```python
from build123d import *

# Parameters (mm, degrees)
SKETCH2_W           = 6.5
SKETCH2_H           = 6.5
BOSS_EXTRUDE1_DEPTH = 8.5
SKETCH4_W           = 15
SKETCH4_H           = 2
BOSS_EXTRUDE2_DEPTH = 15
SKETCH5_R           = 2.7
CUT_EXTRUDE1_DEPTH  = 23.774998804
SKETCH6_W           = 6.5
SKETCH6_H           = 87
BOSS_EXTRUDE3_DEPTH = 2
CUT_EXTRUDE3_DEPTH  = 103.034534305
CUT_EXTRUDE4_DEPTH  = 99.257059971
CUT_EXTRUDE5_DEPTH  = 99.257059971
CUT_EXTRUDE6_DEPTH  = 99.257059971
CUT_EXTRUDE7_DEPTH  = 103.034534305


with BuildPart() as part:
    # Sketch2 → Boss-Extrude1 (new body)
    with BuildSketch(Plane(origin=(0, 0, 0), x_dir=(1, 0, 0), z_dir=(0, 1, 0))):
        with Locations((-0.156417112, 0.017379679)):
            Rectangle(SKETCH2_W, SKETCH2_H)
    extrude(amount=BOSS_EXTRUDE1_DEPTH)

    # Sketch4 → Boss-Extrude2 (add)
    with BuildSketch(Plane.ZY.offset(3.406417112)):
        with Locations((4.232620321, 1)):
            Rectangle(SKETCH4_W, SKETCH4_H)
    extrude(amount=BOSS_EXTRUDE2_DEPTH)

    # Sketch5 → Cut-Extrude1 (cut, through all)
    with BuildSketch(Plane(origin=(0, 2, 0), x_dir=(1, 0, 0), z_dir=(0, 1, 0))):
        with Locations(Location((-10.906417112, -4.232620321, 0), (0, 0, 270))):
            Circle(SKETCH5_R)
    extrude(amount=-CUT_EXTRUDE1_DEPTH, mode=Mode.SUBTRACT)


with BuildPart() as body_2:
    # Mirror3: mirrored copy
    add(part.part.mirror(Plane(origin=(-18.406417112, 0, 11.732620321), x_dir=(1, 0, 0), z_dir=(0, 0, -1))))


with BuildPart() as body_2_1:
    # Body-Move/Copy3: moved
    add(body_2.part.moved(Location((0, 0, 70))))


with BuildPart() as part_1:
    add(part.part)

    add(body_2_1.part)  # Boss-Extrude3 merges body 2
    # Sketch6 → Boss-Extrude3 (add)
    with BuildSketch(Plane(origin=(0, 0, 0), x_dir=(1, 0, 0), z_dir=(0, 1, 0))):
        with Locations((-0.156417112, -46.732620321)):
            Rectangle(SKETCH6_W, SKETCH6_H)
    extrude(amount=BOSS_EXTRUDE3_DEPTH)

    # Sketch10 → Cut-Extrude3 (cut, through all)
    with BuildSketch(Plane(origin=(0, 0, -3.267379679), x_dir=(-1, 0, 0), z_dir=(0, 0, -1))):
        Polygon((-2.443582888, 8.5), (-3.093582888, 7.85), (-3.093582888, 8.5), align=None)
    extrude(amount=-CUT_EXTRUDE3_DEPTH, mode=Mode.SUBTRACT)

    # Sketch7 → Cut-Extrude4 (cut, through all)
    with BuildSketch(Plane.ZY.offset(3.406417112)):
        Polygon((2.582620321, 8.5), (3.232620321, 7.85), (3.232620321, 8.5), align=None)
    extrude(amount=-CUT_EXTRUDE4_DEPTH, mode=Mode.SUBTRACT)

    # Sketch12 → Cut-Extrude5 (cut, through all)
    with BuildSketch(Plane.ZY.offset(3.406417112)):
        Polygon((-2.617379679, 8.5), (-3.267379679, 7.85), (-3.267379679, 8.5), align=None)
    extrude(amount=-CUT_EXTRUDE5_DEPTH, mode=Mode.SUBTRACT)

    # Sketch13 → Cut-Extrude6 (cut, through all)
    with BuildSketch(Plane.ZY.offset(3.406417112)):
        Polygon((90.882620321, 8.5), (90.232620321, 7.85), (90.232620321, 8.5), align=None)
        Polygon((96.082620321, 8.5), (96.732620321, 7.85), (96.732620321, 8.5), align=None)
    extrude(amount=-CUT_EXTRUDE6_DEPTH, mode=Mode.SUBTRACT)

    # Sketch11 → Cut-Extrude7 (cut, through all)
    with BuildSketch(Plane(origin=(0, 0, -3.267379679), x_dir=(-1, 0, 0), z_dir=(0, 0, -1))):
        Polygon((2.756417112, 8.5), (3.406417112, 7.85), (3.406417112, 8.5), align=None)
    extrude(amount=-CUT_EXTRUDE7_DEPTH, mode=Mode.SUBTRACT)


solid = part_1.part
```
Geometry check sheet. Reference: the model listing, model coordinates, mm. A direction names the side the tool comes from. Round coordinates to 2 decimals unless told otherwise and drop trailing zeros. Loops run counter-clockwise (first coordinate to the right, second up) from the corner with the lowest first, then second, coordinate; pieces in that order, holes last. Notation, with made-up numbers: (-38.5, 60.25) - (3.5, 60.25) arc R20 ccw to (3.5, 87.25) - close; hole circle Ø5 at (63, -2). An arc over 180 degrees is marked (long way). Use a Markdown table: item, result.
Q1. Material ranges on line 1 (Z direction, x = -1.5, y = 5.75); line 2 (X direction, y = 1.5, z = 35.5); line 3 (Y direction, x = 1.5, z = 9.5), recorded low to high.
Solutions:
| item | result |
|---|---|
| line 1 | z = -3.27 to 3.23, 90.23 to 96.73 |
| line 2 | x = -3.41 to 3.09 |
| line 3 | y = 0 to 2 |
Q2. Draft check along Z on faces 1 (the flat face through (-3, 3, -3.267)), 2 (the cylindrical face through (-10.79, 1.01, 91.93)), 3 (the flat face through (-3.406, 5, 0)). Enter one of: released by +Z, released by -Z, zero draft, split by the parting line, or undercut.
Solutions:
| item | result |
|---|---|
| face 1 | released by -Z |
| face 2 | undercut |
| face 3 | zero draft |
Q3. Go/stop test with a flat-tipped pin: P1, Ø2, axis at y = 0.5, z = 60, coming from the -X side. Record where the tip stops, or that it passes through.
Solutions:
| item | result |
|---|---|
| P1 | stops at x = -3.41 |
Q4. Cross-section at D-D on x = -10. Record the cut outline in (y, z).
Solutions:
| item | result |
|---|---|
| outline | (0, -3.27) - (2, -3.27) - (2, 1.69) - (0, 1.69) - close; (0, 6.78) - (2, 6.78) - (2, 11.73) - (0, 11.73) - close; (0, 81.73) - (2, 81.73) - (2, 86.69) - (0, 86.69) - close; (0, 91.78) - (2, 91.78) - (2, 96.73) - (0, 96.73) - close |
Q5. Cross-section at C-C on x = 0. Record the cut outline in (y, z).
Solutions:
| item | result |
|---|---|
| outline | (0, -3.27) - (7.85, -3.27) - (8.5, -2.62) - (8.5, 2.58) - (7.85, 3.23) - (2, 3.23) - (2, 90.23) - (7.85, 90.23) - (8.5, 90.88) - (8.5, 96.08) - (7.85, 96.73) - (0, 96.73) - close |
Q6. Cross-section at A-A on x = -5. Record the cut outline in (y, z), plus the area to 3 significant figures.
Solutions:
| item | result |
|---|---|
| outline | (0, -3.27) - (2, -3.27) - (2, 11.73) - (0, 11.73) - close; (0, 81.73) - (2, 81.73) - (2, 96.73) - (0, 96.73) - close |
| area | 60.0 mm2 |
Q7. Access from +Z, -Z, +X, -X, +Y, -Y to the whole of each face (thin tool, end or side, straight path). Record for faces 4 (the flat face through (0, 5, 90.233)), 5 (the flat face through (-3.406, 5, 93)), 6 (the flat face through (-11, 1, 81.733)).
Solutions:
| item | result |
|---|---|
| face 4 | +X, -X, +Y |
| face 5 | +Z, -Z, -X, +Y |
| face 6 | -X, +Y, -Y |
Q8. Cross-section at B-B on y = 3.75. Record the cut outline in (x, z), plus the area to 3 significant figures.
Solutions:
| item | result |
|---|---|
| outline | (-3.41, -3.27) - (3.09, -3.27) - (3.09, 3.23) - (-3.41, 3.23) - close; (-3.41, 90.23) - (3.09, 90.23) - (3.09, 96.73) - (-3.41, 96.73) - close |
| area | 84.5 mm2 |
